Can you work these out from the model? Positions are in its coordinate system, mm. Give positions to 0.01 mm unless a question says otherwise; leave off trailing zeros. Write each loop counter-clockwise with the first axis right and the second up, starting at its lowest first coordinate (ties: lowest second). Pieces come first, ordered by that corner, then holes.
1. Suppose I cut it at A-A (x = 0). Please give me the cut outline in (y, z), and give its area (3 significant figures).
2. If I drill on probe 1 along Z at (x, y) = (38, 3.75); probe 2 along Z at (x, y) = (-1, 4.5); probe 3 along X at (y, z) = (5.25, 3.25), over which ranges is the centre line in solid material (lowest first)?
3. Suppose I cut it at B-B (y = 3.25). Give the number of separate pieces and of enclosed holes in the cut face, and give its area (3 significant figures).
4. I'm going to push a flat-ended pin straight in: pin 1 (1.5 mm diameter, centred on y = 3, z = 3, fed in from +X). Where does the tip first touch, or does it pass through?
```python
from build123d import *

# Parameters (mm, degrees)
SKETCH1_R           = 1.778
BOSS_EXTRUDE1_DEPTH = 6.35


with BuildPart() as part:
    # Sketch1 → Boss-Extrude1 (new body)
    with BuildSketch(Plane(origin=(0, 6.35, 0), x_dir=(1, 0, 0), z_dir=(0, 1, 0))):
        with BuildLine():
            Line((97.79, 4.7625), (-97.79, 4.7625))
            ThreePointArc((-97.79, 4.7625), (-102.5525, 0), (-97.79, -4.7625))
            Line((-97.79, -4.7625), (97.79, -4.7625))
            ThreePointArc((97.79, -4.7625), (102.5525, 0), (97.79, 4.7625))
        make_face()
        with Locations((97.79, 0)):
            Circle(SKETCH1_R, mode=Mode.SUBTRACT)
        with Locations((88.011, 0)):
            Circle(SKETCH1_R, mode=Mode.SUBTRACT)
        with Locations((78.232, 0)):
            Circle(SKETCH1_R, mode=Mode.SUBTRACT)
        with Locations((68.453, 0)):
            Circle(SKETCH1_R, mode=Mode.SUBTRACT)
        with Locations((58.674, 0)):
            Circle(SKETCH1_R, mode=Mode.SUBTRACT)
        with Locations((48.895, 0)):
            Circle(SKETCH1_R, mode=Mode.SUBTRACT)
        with Locations((39.116, 0)):
            Circle(SKETCH1_R, mode=Mode.SUBTRACT)
        with Locations((29.337, 0)):
            Circle(SKETCH1_R, mode=Mode.SUBTRACT)
        with Locations((19.558, 0)):
            Circle(SKETCH1_R, mode=Mode.SUBTRACT)
        with Locations((9.779, 0)):
            Circle(SKETCH1_R, mode=Mode.SUBTRACT)
        Circle(SKETCH1_R, mode=Mode.SUBTRACT)
        with Locations((-9.779, 0)):
            Circle(SKETCH1_R, mode=Mode.SUBTRACT)
        with Locations((-19.558, 0)):
            Circle(SKETCH1_R, mode=Mode.SUBTRACT)
        with Locations((-29.337, 0)):
            Circle(SKETCH1_R, mode=Mode.SUBTRACT)
        with Locations((-39.116, 0)):
            Circle(SKETCH1_R, mode=Mode.SUBTRACT)
        with Locations((-48.895, 0)):
            Circle(SKETCH1_R, mode=Mode.SUBTRACT)
        with Locations((-58.674, 0)):
            Circle(SKETCH1_R, mode=Mode.SUBTRACT)
        with Locations((-68.453, 0)):
            Circle(SKETCH1_R, mode=Mode.SUBTRACT)
        with Locations((-78.232, 0)):
            Circle(SKETCH1_R, mode=Mode.SUBTRACT)
        with Locations((-88.011, 0)):
            Circle(SKETCH1_R, mode=Mode.SUBTRACT)
        with Locations((-97.79, 0)):
            Circle(SKETCH1_R, mode=Mode.SUBTRACT)
    extrude(amount=-BOSS_EXTRUDE1_DEPTH)


solid = part.part
```
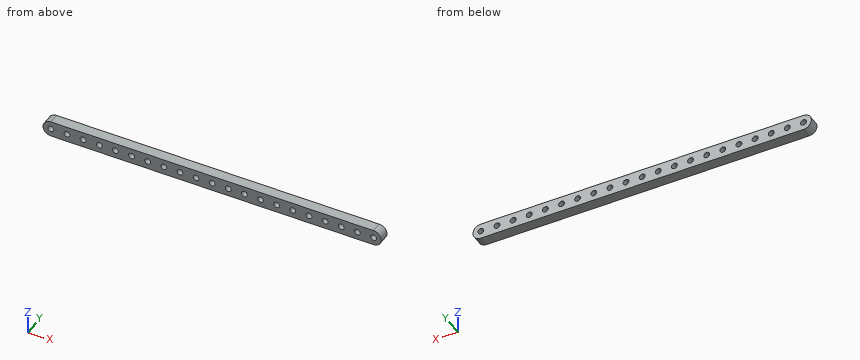
Checks:
1. outline: (0, -4.76) - (6.35, -4.76) - (6.35, -1.78) - (0, -1.78) - close; (0, 1.78) - (6.35, 1.78) - (6.35, 4.76) - (0, 4.76) - close
1. area: 37.9 mm2
2. probe 1: z = -4.76 to -1.38, 1.38 to 4.76
2. probe 2: z = -4.76 to -1.47, 1.47 to 4.76
2. probe 3: x = -101.27 to 101.27
3. separate pieces: 1
3. enclosed holes: 21
3. area: 1,730 mm2
4. pin 1: stops at x = 101.99
